The listing builds one solid part. Answer for the finished solid, in the listing's coordinates (mm). A direction names the side the tool comes from. Give positions to 0.01 mm unless a question says otherwise; leave off trailing zeros. Write each loop counter-clockwise with the first axis right and the second up, starting at its lowest first coordinate (ties: lowest second). Pieces come first, ordered by that corner, then holes. Notation, with made-up numbers: (76, 17.25) -> (122, 17.25) arc R20 ccw to (122, 27.25) -> close; hole circle Ø1 at (29, 51). An arc over 180 degrees is marked (long way). Write each question's results on one line, items separated by ' | '. Start each with the question number.
from build123d import *

# Parameters (mm, degrees)
ESQUISSE2_W     = 10.4
ESQUISSE2_H     = 1.3
FENTE1_DEPTH    = 1.4
ESQUISSE3_W     = 2.5
ESQUISSE3_H     = 13.3
CHANFREIN1_SIZE = 0.5


with BuildPart() as part:
    # Esquisse1 → Base-R_volution (revolve)
    with BuildSketch(Plane(origin=(0, 0, 0), x_dir=(1, 0, 0), z_dir=(0, 1, 0)), mode=Mode.PRIVATE) as base_r_volution_sk:
        Polygon((2.5, 0), (5.2, 2.607359692), (5.2, 2.7), (0, 2.7), (0, 0), align=None)
    revolve(base_r_volution_sk.sketch.rotate(Axis((0, 0, 0), (0, 0, -1)), 180), axis=Axis((0, 0, 0), (0, 0, -1)))

    # Esquisse2 → fente1 (cut)
    with BuildSketch(Plane.XY.offset(-2.7)):
        Rectangle(ESQUISSE2_W, ESQUISSE2_H)
    extrude(amount=FENTE1_DEPTH, mode=Mode.SUBTRACT)

    # Esquisse3 → Boss.-R_vol.1 (revolve)
    with BuildSketch(Plane(origin=(0, 0, 0), x_dir=(1, 0, 0), z_dir=(0, 1, 0)), mode=Mode.PRIVATE) as boss_r_vol_1_sk:
        with Locations((1.25, -6.65)):
            Rectangle(ESQUISSE3_W, ESQUISSE3_H)
    revolve(boss_r_vol_1_sk.sketch.rotate(Axis((0, 0, 0), (0, 0, 1)), 172.819244219), axis=Axis((0, 0, 0), (0, 0, 1)))

    # Chanfrein1
    chanfrein1_edges = [part.edges().sort_by_distance(p)[0] for p in [
        (2.480391854, -0.3125, 13.3),
    ]]
    chamfer(chanfrein1_edges, length=CHANFREIN1_SIZE)


solid = part.part
1. Section A-A (x = 0) is taken. Write down the section's boundary in (y, z).
2. Consider probe 1 along Y at (x, z) = (-1.5, 7.75); probe 2 along Z at (x, y) = (2.5, 0.75). Determine where each line is inside the solid, lowest interval first. Write a range as [from, to].
3. Each of these flat-tipped pins is pushed along its axis until it touches: pin 1 Ø1.5 at (x, z) = (-1.5, -2) entering from +Y; pin 2 Ø1 at (x, y) = (-3.5, 2.5) entering from +Z; pin 3 Ø1.5 at (y, z) = (-1.5, 8.5) entering from +X. Where does it stop, or does it pass through?
4. Section C-C (z = 10.75) is taken. Write down the section's boundary in (x, y).
5. Section B-B (y = 0) is taken. Write down the section's boundary in (x, z), then the cut area to 3 significant figures.
6. A tool of negligible diameter and unlimited length cuts with its end or side. For faces 1 (the cylindrical face through (0, -2.5, 6.3)), 2 (the flat face through (0, -0.65, -2)), 3 (the flat face through (0, 0, 13.3)), from which of +Z, -Z, +X, -X, +Y, -Y can it reach the whole face along a straight path? Write none if from no direction.
Results:
1) outline: (-5.2, -2.7) -> (-0.65, -2.7) -> (-0.65, -1.3) -> (0.65, -1.3) -> (0.65, -2.7) -> (5.2, -2.7) -> (5.2, -2.61) -> (2.5, 0) -> (2.5, 12.8) -> (2, 13.3) -> (-2, 13.3) -> (-2.5, 12.8) -> (-2.5, 0) -> (-5.2, -2.61) -> close
2) probe 1: y = [-2, 2] | probe 2: z = [-2.7, -0.11]
3) pin 1: stops at y = 5.09 | pin 2: stops at z = -1.26 | pin 3: stops at x = 2.38
4) outline: circle Ø5 at (0, 0)
5) outline: (-3.85, -1.3) -> (3.85, -1.3) -> (2.5, 0) -> (2.5, 12.8) -> (2, 13.3) -> (-2, 13.3) -> (-2.5, 12.8) -> (-2.5, 0) -> close | area: 74.5 mm²
6) face 1: +Z | face 2: -Z, +X, -X | face 3: +Z, +X, -X, +Y, -Y
